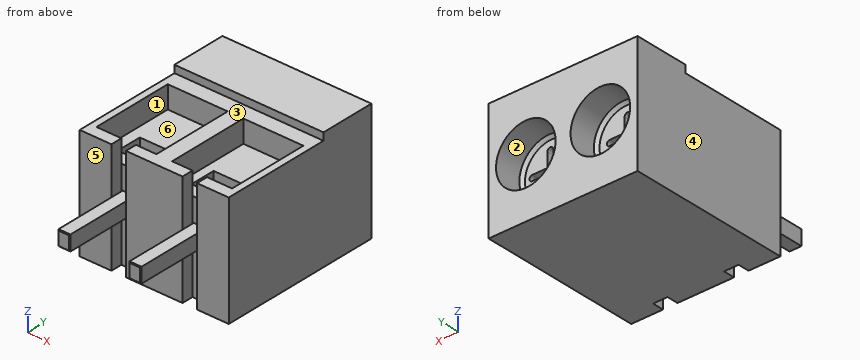
from build123d import *

# Parameters (mm, degrees)
CROQUIS1_W                      = 10
CROQUIS1_H                      = 11
SALIENTE_EXTRUIR1_DEPTH         = 8
CROQUIS2_R                      = 2
CORTAR_EXTRUIR1_DEPTH           = 2
CROQUIS3_W                      = 10
CROQUIS3_H                      = 7.302971928
CORTAR_EXTRUIR2_DEPTH           = 0.5
CROQUIS4_W                      = 4.024100916
CROQUIS4_H                      = 5.499604586
CORTAR_EXTRUIR3_DEPTH           = 1.5
CROQUIS5_W                      = 2.727446176
CROQUIS5_H                      = 1.699064831
CORTAR_EXTRUIR4_DEPTH           = 3.5
CORTAR_EXTRUIR5_DEPTH           = 1
CORTAR_EXTRUIR5_DRAFT           = -3
CORTAR_EXTRUIR5_PROFILE_2_DEPTH = 1
CORTAR_EXTRUIR5_PROFILE_2_DRAFT = -3
CHAFL_N1_SIZE                   = 0.2
CORTAR_EXTRUIR6_DEPTH           = 11.559356041
CROQUIS8_W                      = 0.8
CROQUIS8_H                      = 1.009702069
SALIENTE_EXTRUIR2_DEPTH         = 5
CHAFL_N2_SIZE                   = 0.05


with BuildPart() as part:
    # Croquis1 → Saliente-Extruir1 (new body)
    with BuildSketch(Plane.XY):
        Rectangle(CROQUIS1_W, CROQUIS1_H)
    extrude(amount=SALIENTE_EXTRUIR1_DEPTH)

    # Croquis2 → Cortar-Extruir1 (cut)
    with BuildSketch(Plane(origin=(0, 5.5, 0), x_dir=(1, 0, 0), z_dir=(0, 1, 0))):
        with Locations(Location((2.5, -4, 0), (0, 0, 270))):
            Circle(CROQUIS2_R)
        with Locations(Location((-2.5, -4, 0), (0, 0, 90))):
            Circle(CROQUIS2_R)
    extrude(amount=-CORTAR_EXTRUIR1_DEPTH, mode=Mode.SUBTRACT)

    # Croquis3 → Cortar-Extruir2 (cut)
    with BuildSketch(Plane.XY.offset(8)):
        with Locations((0, -1.848514036)):
            Rectangle(CROQUIS3_W, CROQUIS3_H)
    extrude(amount=-CORTAR_EXTRUIR2_DEPTH, mode=Mode.SUBTRACT)

    # Croquis4 → Cortar-Extruir3 (cut)
    with BuildSketch(Plane.XY.offset(7.5)):
        with Locations((-2.537419189, -1.978516284)):
            Rectangle(CROQUIS4_W, CROQUIS4_H)
        with Locations((2.537419189, -1.978516284)):
            Rectangle(CROQUIS4_W, CROQUIS4_H)
    extrude(amount=-CORTAR_EXTRUIR3_DEPTH, mode=Mode.SUBTRACT)

    # Croquis5 → Cortar-Extruir4 (cut)
    with BuildSketch(Plane.XY.offset(6)):
        with Locations((-2.474433562, -3.051609862)):
            Rectangle(CROQUIS5_W, CROQUIS5_H)
        with Locations((2.474433562, -3.051609862)):
            Rectangle(CROQUIS5_W, CROQUIS5_H)
    extrude(amount=-CORTAR_EXTRUIR4_DEPTH, mode=Mode.SUBTRACT)


with BuildPart() as cortar_extruir5_tool:
    # Croquis6 → Cortar-Extruir5 (with draft: the straight prism first)
    with BuildSketch(Plane(origin=(0, 3.5, 0), x_dir=(1, 0, 0), z_dir=(0, 1, 0))):
        with BuildLine():
            Line((-2.796040432, -4.215779763), (-2.796040432, -5.17015319))
            ThreePointArc((-2.796040432, -5.17015319), (-2.592982256, -5.373211365), (-2.38992408, -5.17015319))
            Line((-2.38992408, -5.17015319), (-2.38992408, -4.215779763))
            Line((-2.38992408, -4.215779763), (-1.374633201, -4.215779763))
            ThreePointArc((-1.374633201, -4.215779763), (-1.191880843, -4.033027405), (-1.374633201, -3.850275046))
            Line((-1.374633201, -3.850275046), (-2.38992408, -3.850275046))
            Line((-2.38992408, -3.850275046), (-2.38992408, -2.89590162))
            ThreePointArc((-2.38992408, -2.89590162), (-2.592982256, -2.692843444), (-2.796040432, -2.89590162))
            Line((-2.796040432, -2.89590162), (-2.796040432, -3.850275046))
            Line((-2.796040432, -3.850275046), (-3.811331312, -3.850275046))
            ThreePointArc((-3.811331312, -3.850275046), (-3.99408367, -4.033027405), (-3.811331312, -4.215779763))
            Line((-3.811331312, -4.215779763), (-2.796040432, -4.215779763))
        make_face()
    extrude(amount=-CORTAR_EXTRUIR5_DEPTH)
    # Cortar-Extruir5: the draft: its side faces are tilted about the plane it starts from
    cortar_extruir5_sides = [cortar_extruir5_tool.faces().sort_by_distance(p)[0] for p in [
        (-2.796040432, 3, 3.373088333),
        (-3.303685872, 3, 3.850275046),
        (-3.99408367, 3, 4.033027405),
        (-3.303685872, 3, 4.215779763),
        (-2.796040432, 3, 4.692966476),
        (-2.592982256, 3, 5.373211365),
        (-2.38992408, 3, 4.692966476),
        (-1.882278641, 3, 4.215779763),
        (-1.191880843, 3, 4.033027405),
        (-1.882278641, 3, 3.850275046),
        (-2.38992408, 3, 3.373088333),
        (-2.592982256, 3, 2.692843444),
    ]]
    draft(cortar_extruir5_sides, Plane(origin=(0, 3.5, 0), x_dir=(1, 0, 0), z_dir=(0, 1, 0)), CORTAR_EXTRUIR5_DRAFT)


with BuildPart() as part_1:
    add(part.part)

    # Cortar-Extruir5: cut by cortar_extruir5_tool
    add(cortar_extruir5_tool.part, mode=Mode.SUBTRACT)


with BuildPart() as cortar_extruir5_profile_2_tool:
    # Croquis6 → Cortar-Extruir5 profile 2 (with draft: the straight prism first)
    with BuildSketch(Plane(origin=(0, 3.5, 0), x_dir=(1, 0, 0), z_dir=(0, 1, 0))):
        with BuildLine():
            Line((2.38992408, -4.215779763), (2.38992408, -5.17015319))
            ThreePointArc((2.38992408, -5.17015319), (2.592982256, -5.373211365), (2.796040432, -5.17015319))
            Line((2.796040432, -5.17015319), (2.796040432, -4.215779763))
            Line((2.796040432, -4.215779763), (3.811331312, -4.215779763))
            ThreePointArc((3.811331312, -4.215779763), (3.99408367, -4.033027405), (3.811331312, -3.850275046))
            Line((3.811331312, -3.850275046), (2.796040432, -3.850275046))
            Line((2.796040432, -3.850275046), (2.796040432, -2.89590162))
            ThreePointArc((2.796040432, -2.89590162), (2.592982256, -2.692843444), (2.38992408, -2.89590162))
            Line((2.38992408, -2.89590162), (2.38992408, -3.850275046))
            Line((2.38992408, -3.850275046), (1.374633201, -3.850275046))
            ThreePointArc((1.374633201, -3.850275046), (1.191880843, -4.033027405), (1.374633201, -4.215779763))
            Line((1.374633201, -4.215779763), (2.38992408, -4.215779763))
        make_face()
    extrude(amount=-CORTAR_EXTRUIR5_PROFILE_2_DEPTH)
    # Cortar-Extruir5 profile 2: the draft: its side faces are tilted about the plane it starts from
    cortar_extruir5_profile_2_sides = [cortar_extruir5_profile_2_tool.faces().sort_by_distance(p)[0] for p in [
        (2.38992408, 3, 4.692966476),
        (2.592982256, 3, 5.373211365),
        (2.796040432, 3, 4.692966476),
        (3.303685872, 3, 4.215779763),
        (3.99408367, 3, 4.033027405),
        (3.303685872, 3, 3.850275046),
        (2.796040432, 3, 3.373088333),
        (2.592982256, 3, 2.692843444),
        (2.38992408, 3, 3.373088333),
        (1.882278641, 3, 3.850275046),
        (1.191880843, 3, 4.033027405),
        (1.882278641, 3, 4.215779763),
    ]]
    draft(cortar_extruir5_profile_2_sides, Plane(origin=(0, 3.5, 0), x_dir=(1, 0, 0), z_dir=(0, 1, 0)), CORTAR_EXTRUIR5_PROFILE_2_DRAFT)


with BuildPart() as part_2:
    add(part_1.part)

    # Cortar-Extruir5 profile 2: cut by cortar_extruir5_profile_2_tool
    add(cortar_extruir5_profile_2_tool.part, mode=Mode.SUBTRACT)

    # Chaflán1
    chafl_n1_edges = [part_2.edges().sort_by_distance(p)[0] for p in [
        (2.5, 3.5, 2),
        (-2.5, 3.5, 6),
    ]]
    chamfer(chafl_n1_edges, length=CHAFL_N1_SIZE)

    # Croquis7 → Cortar-Extruir6 (cut, through all)
    with BuildSketch(Plane.XY.offset(7.5)):
        Polygon((-2.869109202, -5.079330001), (-2.869109202, -5.629900541), (-1.898102979, -5.629900541), (-1.898102979, -5.079330001), (-1.898102979, -4.728318577), (-2.869109202, -4.728318577), align=None)
        Polygon((2.869109202, -4.728318577), (2.869109202, -5.079330001), (2.869109202, -5.629900541), (1.898102979, -5.629900541), (1.898102979, -5.079330001), (1.898102979, -4.728318577), align=None)
    extrude(amount=-CORTAR_EXTRUIR6_DEPTH, mode=Mode.SUBTRACT)

    # Croquis8 → Saliente-Extruir2 (add)
    with BuildSketch(Plane.XZ.offset(4.728318577)):
        with Locations((-2.383102979, 3.926715173)):
            Rectangle(CROQUIS8_W, CROQUIS8_H)
        with Locations((2.383102979, 3.926715173)):
            Rectangle(CROQUIS8_W, CROQUIS8_H)
    extrude(amount=SALIENTE_EXTRUIR2_DEPTH)

    # Chaflán2
    chafl_n2_edges = [part_2.edges().sort_by_distance(p)[0] for p in [
        (-1.983102979, -9.728318577, 3.926715172),
        (-2.383102979, -9.728318577, 4.431566207),
        (-2.783102979, -9.728318577, 3.926715172),
        (-2.383102979, -9.728318577, 3.421864138),
        (2.783102979, -9.728318577, 3.926715172),
        (2.383102979, -9.728318577, 4.431566207),
        (1.983102979, -9.728318577, 3.926715172),
        (2.383102979, -9.728318577, 3.421864138),
    ]]
    chamfer(chafl_n2_edges, length=CHAFL_N2_SIZE)


solid = part_2.part
For this review, take the finished solid that the model builds, in its own axes (mm). Face numbers are marked on the shaded views. A direction names the side the tool comes from. Give positions to 0.01 mm unless a question says otherwise; leave off trailing zeros. Loops run counter-clockwise (first coordinate to the right, second up) from the corner with the lowest first, then second, coordinate; pieces in that order, holes last. Notation, with made-up numbers: M -14.75,46.5 L -4.75,46.5 A19 ccw -4.75,74.5 Z; hole C 27,68.5 d10. An arc over 180 degrees is marked long. Put each result on its own line as item: value. Start each with the question number.
(1) Wall thickness on L1, parallel to X at y = 4.75, z = 4; L2, parallel to X at y = -5, z = 1.25; L3, parallel to Y at x = 3.75, z = 5.75: over which ranges is each line inside the solid? List them lowest first.
(2) Machinability: for the marked faces 1, 2 and 3, which of the approach directions +Z, -Z, +X, -X, +Y, -Y give a long, thin tool a straight path to every point of the face, cutting with its end or side? Answer none if there is none.
(3) Add section C-C, the plane z = 1.25. Write out the cut boundary in (x, y), then the cut area to 3 significant figures.
(4) The part is to be moulded in two halves that separate along X. For the marked faces 4, 5 and 6, say which applies: +X half, -X half, draft (parallel to the pull), parting line (faces both ways), or undercut.
(5) Add section A-A, the plane z = 7.25. Write out the cut boundary in (x, y).
(6) For pin 1 (0.6 mm diameter, centred on x = 2.5, y = -7.5, fed in from +Z); pin 2 (2 mm diameter, centred on x = 3.5, y = -8, fed in from -Z); pin 3 (0.8 mm diameter, centred on x = 2, z = 6.5, fed in from -Y), all flat-tipped, find the tip position at first contact; note any pin that passes through.
(7) Add section D-D, the plane y = -3.25. Write out the cut boundary in (x, z).
(8) Add section B-B, the plane y = 0.5. Write out the cut boundary in (x, z).
Result:
1. L1: x = -5 to -4.5, -0.5 to 0.5, 4.5 to 5
1. L2: x = -5 to -2.87, -1.9 to 1.9, 2.87 to 5
1. L3: y = -5.5 to -3.9, -2.2 to 5.5
2. face 1: +Z
2. face 2: +Y
2. face 3: +Z, +X, -X, -Y
3. outline: M -5,-5.5 L -2.87,-5.5 L -2.87,-4.73 L -1.9,-4.73 L -1.9,-5.5 L 1.9,-5.5 L 1.9,-4.73 L 2.87,-4.73 L 2.87,-5.5 L 5,-5.5 L 5,5.5 L -5,5.5 Z
3. area: 109 mm^2
4. face 4: -X half
4. face 5: draft
4. face 6: undercut
5. outline: M -5,-5.5 L -2.87,-5.5 L -2.87,-4.73 L -4.55,-4.73 L -4.55,0.77 L -0.53,0.77 L -0.53,-4.73 L -1.9,-4.73 L -1.9,-5.5 L 1.9,-5.5 L 1.9,-4.73 L 0.53,-4.73 L 0.53,0.77 L 4.55,0.77 L 4.55,-4.73 L 2.87,-4.73 L 2.87,-5.5 L 5,-5.5 L 5,5.5 L -5,5.5 Z
6. pin 1: stops at z = 4.43
6. pin 2: stops at z = 3.42
6. pin 3: stops at y = -5.5
7. outline: M -5,0 L 5,0 L 5,7.5 L 4.55,7.5 L 4.55,6 L 3.84,6 L 3.84,2.5 L 1.11,2.5 L 1.11,6 L 0.53,6 L 0.53,7.5 L -0.53,7.5 L -0.53,6 L -1.11,6 L -1.11,2.5 L -3.84,2.5 L -3.84,6 L -4.55,6 L -4.55,7.5 L -5,7.5 Z
8. outline: M -5,0 L 5,0 L 5,7.5 L 4.55,7.5 L 4.55,6 L 0.53,6 L 0.53,7.5 L -0.53,7.5 L -0.53,6 L -4.55,6 L -4.55,7.5 L -5,7.5 Z
